Here's how the part is built. I have some questions about the finished solid (model axes, mm). Face numbers are marked on the shaded views. Coordinates: 2 decimals unless noted, no trailing zeros. Write each loop counter-clockwise with the first axis right and the second up, starting at its lowest first coordinate (ties: lowest second). Pieces come first, ordered by that corner, then holes. Notation, with made-up numbers: (55.25, 80.5) -> (65.25, 80.5) arc R18 cw to (65.25, 95.5) -> close; hole circle Ø8 at (6.5, 7). An arc over 180 degrees is marked (long way). Put each result on its own line as item: value. Start each with the question number.
Item 1: I want a section at B-B, the plane x = 4.15. List the corners of the cut face in (y, z) for me.
Item 2: I want a section at A-A, the plane y = -0.85. List the corners of the cut face in (x, z) for me.
Item 3: I want a section at C-C, the plane x = -1.75. List the corners of the cut face in (y, z) for me.
Item 4: I need wall thicknesses on line 1 (Z direction, x = 1.25, y = -1.15) (3 decimals); line 2 (Z direction, x = -3.75, y = 1.2). Which ranges of each line are inside material? Lowest first, please. Write a range as [from, to].
Item 5: If we mould it in two halves opening along X, with no side actions, what happens to the marked faces 1, 2, 3 and 4? For each: released by +X, released by -X, zero draft, split by the parting line, or undercut.
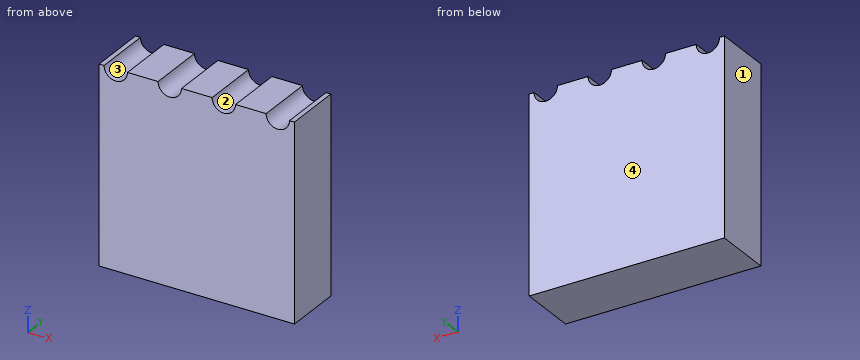
from build123d import *

# Parameters (mm, degrees)
SKETCH1_W           = 10
SKETCH1_H           = 10
BOSS_EXTRUDE1_DEPTH = 1.5
CUT_EXTRUDE1_DEPTH  = 1.5
LPATTERN1_COUNT     = 4
LPATTERN1_PITCH     = 2.766666667


with BuildPart() as part:
    # Sketch1 → Boss-Extrude1 (new body, symmetric)
    with BuildSketch(Plane(origin=(0, 0, 0), x_dir=(1, 0, 0), z_dir=(0, 1, 0))):
        Rectangle(SKETCH1_W, SKETCH1_H)
    extrude(amount=BOSS_EXTRUDE1_DEPTH, both=True)

    # Sketch2 → Cut-Extrude1 (cut, symmetric)
    with BuildSketch(Plane(origin=(0, 0, 0), x_dir=(1, 0, 0), z_dir=(0, 1, 0))):
        with BuildLine():
            Line((-4.75, -5), (-3.55, -5))
            ThreePointArc((-3.55, -5), (-4.15, -4.4), (-4.75, -5))
        make_face()
    cut_extrude1 = extrude(amount=CUT_EXTRUDE1_DEPTH, both=True, mode=Mode.SUBTRACT)

    # LPattern1: Cut-Extrude1 ×4
    with Locations(*[(i * LPATTERN1_PITCH, 0, 0) for i in range(1, LPATTERN1_COUNT)]):
        add(cut_extrude1, mode=Mode.SUBTRACT)


solid = part.part
Calculated:
1. outline: (-1.5, -5) -> (1.5, -5) -> (1.5, 4.4) -> (-1.5, 4.4) -> close
2. outline: (-5, -5) -> (5, -5) -> (5, 5) -> (4.75, 5) arc R0.6 cw to (3.55, 5) -> (1.98, 5) arc R0.6 cw to (0.78, 5) -> (-0.78, 5) arc R0.6 cw to (-1.98, 5) -> (-3.55, 5) arc R0.6 cw to (-4.75, 5) -> (-5, 5) -> close
3. outline: (-1.5, -5) -> (1.5, -5) -> (1.5, 4.53) -> (-1.5, 4.53) -> close
4. line 1: z = [-5, 4.415]
4. line 2: z = [-5, 4.55]
5. face 1: released by -X
5. face 2: undercut
5. face 3: undercut
5. face 4: zero draft
